Here's how the part is built. I have some questions about the finished solid (model axes, mm). Coordinates: 2 decimals unless noted, no trailing zeros. Write each loop counter-clockwise with the first axis right and the second up, starting at its lowest first coordinate (ties: lowest second). Pieces come first, ordered by that corner, then holes. Notation, with made-up numbers: (-33, 20.5) -> (-1, 20.5) arc R16 ccw to (-1, 51.5) -> close; hole circle Ø4 at (-7, 14). An arc over 180 degrees is marked (long way). Answer in a Markdown table with one row per item. Add a question column.
from build123d import *

# Parameters (mm, degrees)
SALIENTE_EXTRUIR1_DEPTH = 1.5
CROQUIS2_R              = 2.5
CORTAR_EXTRUIR1_DEPTH   = 1.4


with BuildPart() as part:
    # Croquis1 → Saliente-Extruir1 (new body)
    with BuildSketch(Plane.XY):
        with BuildLine():
            Line((-47.708333333, 74.739583333), (62.291666667, 74.739583333))
            ThreePointArc((62.291666667, 74.739583333), (76.43380229, 68.881718957), (82.291666667, 54.739583333))
            Line((82.291666667, 54.739583333), (82.291666667, -85.260416667))
            ThreePointArc((82.291666667, -85.260416667), (76.43380229, -99.40255229), (62.291666667, -105.260416667))
            Line((62.291666667, -105.260416667), (-47.708333333, -105.260416667))
            ThreePointArc((-47.708333333, -105.260416667), (-61.850468957, -99.40255229), (-67.708333333, -85.260416667))
            Line((-67.708333333, -85.260416667), (-67.708333333, 54.739583333))
            ThreePointArc((-67.708333333, 54.739583333), (-61.850468957, 68.881718957), (-47.708333333, 74.739583333))
        make_face()
    extrude(amount=SALIENTE_EXTRUIR1_DEPTH)

    # Croquis2 → Cortar-Extruir1 (cut)
    with BuildSketch(Plane(origin=(0, 0, 0), x_dir=(-1, 0, 0), z_dir=(0, 0, -1))):
        with Locations((-47.791666667, 45.239583333)):
            Circle(CROQUIS2_R)
        with Locations((33.208333333, 45.239583333)):
            Circle(CROQUIS2_R)
        with Locations((33.208333333, -75.760416667)):
            Circle(CROQUIS2_R)
        with Locations((-47.791666667, -75.760416667)):
            Circle(CROQUIS2_R)
    extrude(amount=-CORTAR_EXTRUIR1_DEPTH, mode=Mode.SUBTRACT)


solid = part.part
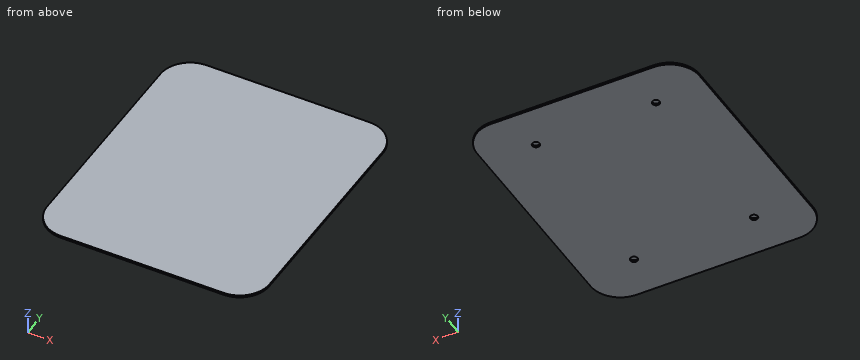
Q1. I'm going to push a flat-ended pin straight in: P1, Ø1.5, axis at x = -33, y = 45.5, coming from the -Z side. Where does the tip first touch, or does it pass through?
Q2. I need wall thicknesses on line 1 (X direction, y = 45, z = 1.3); line 2 (Y direction, x = 70.5, z = 0.1); line 3 (Y direction, x = -54.5, z = 0.2). Which ranges of each line are inside material? Lowest first, please. Write a range as [from, to].
Q3. Imagine slicing it at B-B on x = 70. Please give me the cut outline in (y, z), plus the area to 3 significant figures.
Q4. Imagine slicing it at A-A on z = 0.5. Please give me the cut outline in (x, y), plus the area to 3 significant figures.
Result sheet:
| question | item | result |
|---|---|---|
| 1 | P1 | stops at z = 1.4 |
| 2 | line 1 | x = [-67.71, -35.7], [-30.72, 45.3], [50.28, 82.29] |
| 2 | line 2 | y = [-103.5, 72.98] |
| 2 | line 3 | y = [-104.07, 73.55] |
| 3 | outline | (-103.72, 0) -> (73.19, 0) -> (73.19, 1.5) -> (-103.72, 1.5) -> close |
| 3 | area | 265 mm^2 |
| 4 | outline | (-67.71, -85.26) arc R20 ccw to (-47.71, -105.26) -> (62.29, -105.26) arc R20 ccw to (82.29, -85.26) -> (82.29, 54.74) arc R20 ccw to (62.29, 74.74) -> (-47.71, 74.74) arc R20 ccw to (-67.71, 54.74) -> close; hole circle Ø5 at (-33.21, -75.76); hole circle Ø5 at (-33.21, 45.24); hole circle Ø5 at (47.79, -75.76); hole circle Ø5 at (47.79, 45.24) |
| 4 | area | 26,600 mm^2 |
